The model under review builds one solid part; all positions refer to its coordinate system, in mm. A direction names the side the tool comes from. Coordinates: 2 decimals unless noted, no trailing zeros. Order: outer loops, then holes, each group sorted by start corner. A loop starts at its lowest first (then second) coordinate and runs counter-clockwise, first axis right, second up. Notation, with made-up numbers: (63.5, 23) -> (79.5, 23) arc R15 cw to (79.5, 50) -> close; hole circle Ø9 at (55, 15). An arc over 180 degrees is marked (long way). Use CSV: the item, a comma, the result in double quotes. Start each with the question number.
```python
from build123d import *

# Parameters (mm, degrees)
BOSS_EXTRUDE1_DEPTH     = 90
CUT_EXTRUDE1_DEPTH      = 221.737400712
CUT_EXTRUDE1_DEPTH_BACK = 221.737400712
SKETCH3_R               = 6
CUT_EXTRUDE2_DEPTH      = 203.489832762
CUT_EXTRUDE2_DEPTH_BACK = 203.489832762
SKETCH4_R               = 6
FILLET1_R               = 5
BOSS_EXTRUDE2_DEPTH     = 90
SAVE_BODIES1_DEPTH      = 90


# Read off the part's stored shape, not the designer's step: Save Bodies1
with BuildPart() as part:
    # Sketch1 → Boss-Extrude1 (new body)
    with BuildSketch(Plane(origin=(0, 0, 0), x_dir=(1, 0, 0), z_dir=(0, 1, 0))):
        with BuildLine():
            Line((154.751233709, -116.19), (40, -116.19))
            Line((40, -116.19), (40, -120))
            Line((40, -120), (155.92492368, -120))
            add(Edge.make_bspline(
                [(155.92492368, -120), (169.759222072, -120), (170.545338761, -105)],
                knots=[0, 0, 0, 1.513941954, 1.513941954, 1.513941954], degree=2, weights=[1, 0.726919441, 1]))
            Line((170.545338761, -105), (175, -20))
            Line((175, -20), (171.19, -20))
            Line((171.19, -20), (166.735338761, -105))
            add(Edge.make_bspline(
                [(154.751233709, -116.19), (166.148895711, -116.19), (166.735338761, -105)],
                knots=[1.570796327, 1.570796327, 1.570796327, 3.090116999, 3.090116999, 3.090116999], degree=2, weights=[1, 0.725069971, 1]))
        make_face()
    extrude(amount=BOSS_EXTRUDE1_DEPTH)

    # Sketch3 → Cut-Extrude1 (cut, two sides: drawn at the far end of the back side and taken through both)
    with BuildSketch(Plane.XY.offset(120).offset(-CUT_EXTRUDE1_DEPTH_BACK)):
        with Locations((55, 70)):
            Circle(SKETCH3_R)
        with Locations((55, 20)):
            Circle(SKETCH3_R)
    extrude(amount=CUT_EXTRUDE1_DEPTH + CUT_EXTRUDE1_DEPTH_BACK, mode=Mode.SUBTRACT)

    # Sketch4 → Cut-Extrude2 (cut, two sides: drawn at the far end of the back side and taken through both)
    with BuildSketch(Plane(origin=(176.046719125, 0, 0.027409305), x_dir=(0.052335956242940504, 0, -0.9986295347545742), z_dir=(0.9986295347545742, 0, 0.052335956242940504)).offset(-CUT_EXTRUDE2_DEPTH_BACK)):
        with Locations((-35, 70)):
            Circle(SKETCH4_R)
        with Locations((-35, 20)):
            Circle(SKETCH4_R)
    extrude(amount=CUT_EXTRUDE2_DEPTH + CUT_EXTRUDE2_DEPTH_BACK, mode=Mode.SUBTRACT)

    # Fillet1
    fillet1_edges = [part.edges().sort_by_distance(p)[0] for p in [
        (173.095, 0, 20),
        (173.095, 90, 20),
        (40, 90, 118.095),
        (40, 0, 118.095),
    ]]
    fillet(fillet1_edges, radius=FILLET1_R)


with BuildPart() as body_2:
    # Sketch5 → Boss-Extrude2 (new body)
    with BuildSketch(Plane(origin=(0, 0, 0), x_dir=(1, 0, 0), z_dir=(0, 1, 0))):
        with BuildLine():
            Line((154.751233709, -116.19), (40, -116.19))
            Line((40, -116.19), (40, -96.19))
            Line((40, -96.19), (128.217759962, -96.19))
            ThreePointArc((128.217759962, -96.19), (141.984851476, -90.69748742), (148.190350657, -77.236719125))
            Line((148.190350657, -77.236719125), (151.19, -20))
            Line((151.19, -20), (171.19, -20))
            Line((171.19, -20), (166.735338761, -105))
            add(Edge.make_bspline(
                [(154.751233709, -116.19), (166.148895711, -116.19), (166.735338761, -105)],
                knots=[1.570796327, 1.570796327, 1.570796327, 3.090116999, 3.090116999, 3.090116999], degree=2, weights=[1, 0.725069971, 1]))
        make_face()
    extrude(amount=BOSS_EXTRUDE2_DEPTH)

    # Save Bodies1 outline → Save Bodies1 (cut)
    with BuildSketch(Plane(origin=(0, 0, 0), x_dir=(1, 0, 0), z_dir=(0, 1, 0))):
        with BuildLine():
            Line((171.19, -20), (151.19, -20))
            Line((151.19, -20), (148.190350657, -77.236719125))
            ThreePointArc((148.190350657, -77.236719125), (141.984851476, -90.69748742), (128.217759962, -96.19))
            Line((128.217759962, -96.19), (40, -96.19))
            Line((40, -96.19), (40, -116.19))
            Line((40, -116.19), (154.751233709, -116.19))
            add(Edge.make_bspline(
                [(166.735338761, -105), (166.148895711, -116.19), (154.751233709, -116.19)],
                knots=[3.193068309, 3.193068309, 3.193068309, 4.71238898, 4.71238898, 4.71238898], degree=2, weights=[1, 0.725069971, 1]))
            Line((166.735338761, -105), (171.19, -20))
        make_face()
    extrude(amount=SAVE_BODIES1_DEPTH, mode=Mode.SUBTRACT)


solid = part.part
```
Q1. Clearance check with flat-ended pins moving along their axes: pin 1 Ø19 at (x, y) = (55, 20) entering from -Z; pin 2 Ø5 at (y, z) = (58, 52.5) entering from -X; pin 3 Ø2 at (y, z) = (73, 102.5) entering from -X; pin 4 Ø10 at (x, y) = (156, 12.5) entering from +Z. State where each tip first meets the part, or that it passes through.
Q2. For faces 1 (the cylindrical face through (172.25, 75.95, 35.66)), 2 (the flat face through (98, 44, 116.19)), list the 3-axis set-ups (+Z, -Z, +X, -X, +Y, -Y) from which the entire face can be reached by the end or side of a thin tool; tool diameter is ignored.
Q3. Draft analysis for pull direction Z (two halves, no side actions). For faces 3 (the cylindrical face through (50.58, 74.06, 118.07)), 4 (the flat face through (97, 44, 120)), 5 (the cylindrical face through (172.588, 21.802, 29.163)), state which applies: +Z half, -Z half, draft (parallel to the pull), parting line (faces both ways), or undercut.
Q4. Add section B-B, the plane x = 146. State the section outline as (y, z) points, then the cut area to 3 significant figures.
Q5. Add section A-A, the plane x = 55. State the section outline as (y, z) points, then the cut area to 3 significant figures.
Q6. Add section D-D, the plane z = 91.5. State the section outline as (x, y) points.
Q7. Add section C-C, the plane y = 22.5. State how many separate pieces and enclosed holes the cut face has, then the cut area to 3 significant figures.
Q8. To check wall thickness, follow probe 1 along Z at (x, y) = (117, 62.5); probe 2 along X at (y, z) = (70, 118.2); probe 3 along X at (y, z) = (20, 118). State the ranges of each line that lie inside material, in increasing order.
Answer block:
1,pin 1,"stops at z = 116.19"
1,pin 2,"stops at x = 169.36"
1,pin 3,"stops at x = 166.81"
1,pin 4,"stops at z = 120"
2,face 1,"none"
2,face 2,"-Z, -X, +Y, -Y"
3,face 3,"draft"
3,face 4,"+Z half"
3,face 5,"undercut"
4,outline,"(0, 116.19) -> (90, 116.19) -> (90, 120) -> (0, 120) -> close"
4,area,"343 mm²"
5,outline,"(0, 116.19) -> (14, 116.19) -> (14, 120) -> (0, 120) -> close; (26, 116.19) -> (64, 116.19) -> (64, 120) -> (26, 120) -> close; (76, 116.19) -> (90, 116.19) -> (90, 120) -> (76, 120) -> close"
5,area,"251 mm²"
6,outline,"(167.44, 0) -> (171.25, 0) -> (171.25, 90) -> (167.44, 90) -> close"
7,separate pieces,"3"
7,enclosed holes,"0"
7,area,"761 mm²"
8,probe 1,"z = 116.19 to 120"
8,probe 2,"x = 40 to 49, 61 to 162.69"
8,probe 3,"x = 40 to 49, 61 to 163.03"
